Here's how the part is built. I have some questions about the finished solid (model axes, mm). A direction names the side the tool comes from. Round coordinates to 2 decimals unless told otherwise and drop trailing zeros. Write each loop counter-clockwise with the first axis right and the second up, starting at its lowest first coordinate (ties: lowest second). Pieces come first, ordered by that corner, then holes. Notation, with made-up numbers: M 28,39.5 L 47,39.5 A10 ccw 47,51.5 Z; hole C -29,38.25 d10. An arc over 180 degrees is marked long. Use one line per item in the form item = value. Start each with the question number.
Q1. We'd pull the mould along Z, two halves only. Please class faces 1 (the face through (-9.337, -0.411, 25.38)), 2 (the face through (0, 0, 52.338)), 3 (the face through (1, -1, 0)): +Z half, -Z half, draft (parallel to the pull), parting line (faces both ways), or undercut.
Q2. I want a section at A-A on z = 28.5. List the corners of the cut face in (x, y) for me, and give its area (3 significant figures).
Q3. I want a section at B-B on z = 3. List the corners of the cut face in (x, y) for me, and give its area (3 significant figures).
Q4. For faces 4 (the face through (11.01, 0, 40)), 5 (the face through (-1, 18, 5)), which set-ups out of +Z, -Z, +X, -X, +Y, -Y let a thin tool reach every point of the face, with its end or its side?
Q5. I need wall thicknesses on line 1 along Z through (x, y) = (-1, -38); line 2 along Y through (x, z) = (3.5, 25.5); line 3 along Y through (x, z) = (2, 15). Which ranges of each line are inside material? Lowest first, please. Write a range as from..to.
Q6. I'm going to push flat-ended pins straight in: pin 1 Ø12 at (y, z) = (-1.5, 26) entering from +X; pin 2 Ø2 at (x, z) = (2.5, 15.5) entering from -Y; pin 3 Ø3 at (x, y) = (25, -15) entering from +Z; pin 4 Ø10 at (x, z) = (32, 13) entering from -Y. Where does each tip first touch, or does it pass through?
```python
from build123d import *

# Parameters (mm, degrees)
F3_W     = 13.993276
F3_H     = 39.785632
F4_DEPTH = 25
F5_W     = 45.990731
F5_H     = 9.154398
F6_DEPTH = 12.5
F7_R     = 3


with BuildPart() as f1:
    # F0 (on Front) → F1 (revolve)
    with BuildSketch(Plane.XZ):
        with BuildLine():
            Line((0, 55), (0, 0))
            Line((0, 0), (44, 0))
            Line((44, 0), (40.892728, 5))
            Line((40.892728, 5), (16.228148, 5))
            ThreePointArc((16.228148, 5), (8.850146, 8.601889), (7.152097, 16.634642))
            Line((7.152097, 16.634642), (12.695047, 38.726145))
            ThreePointArc((12.695047, 38.726145), (10.319915, 49.961889), (0, 55))
        make_face()
    revolve(axis=Axis((0, 0, 14.176942), (0, 0, -1)))

    # F3 (on offset) → F4 (cut)
    with BuildSketch(Plane.XY.offset(56)):
        with Locations((18.006259, -3.923812)):
            Rectangle(F3_W, F3_H)
    extrude(amount=-F4_DEPTH, mode=Mode.SUBTRACT)

    # F5 (on Front) → F6 (cut, symmetric)
    with BuildSketch(Plane.XZ):
        with Locations((6.243711, 56.915106)):
            Rectangle(F5_W, F5_H)
    extrude(amount=F6_DEPTH, both=True, mode=Mode.SUBTRACT)

    # F7
    f7_edges = [f1.edges().sort_by_distance(p)[0] for p in [
        (-7.911964, 0, 52.337907),
        (11.009621, -6.026784, 45.623109),
        (11.009621, 6.026784, 45.623109),
        (11.009621, -3.847165, 34.610661),
        (11.009621, 3.847165, 34.610661),
    ]]
    fillet(f7_edges, radius=F7_R)


solid = f1.part
```
Reported:
q1.face_1 = undercut
q1.face_2 = +Z half
q1.face_3 = -Z half
q2.outline = C 0,0 d20.26
q2.area = 322 mm^2
q3.outline = C 0,0 d84.27
q3.area = 5,580 mm^2
q4.face_4 = +Z, +X, +Y, -Y
q4.face_5 = +Z
q5.line_1 = 0..5
q5.line_2 = -8.7..8.7
q5.line_3 = -6.6..6.6
q6.pin_1 = 10.97
q6.pin_2 = -6.83
q6.pin_3 = 5
q6.pin_4 = through
